from build123d import *

# Parameters (mm, degrees)
F0_R     = 6.25
F1_DEPTH = 8


with BuildPart() as f1:
    # F0 (on Top) → F1 (new body)
    with BuildSketch(Plane.XY):
        Polygon((9.494796, -5.493831), (9.505195, 5.475819), (0.010399, 10.96965), (-9.494796, 5.493831), (-9.505195, -5.475819), (-0.010399, -10.96965), align=None)
        Circle(F0_R, mode=Mode.SUBTRACT)
    extrude(amount=F1_DEPTH)

    # F2 (on Right) → F3 (revolve)
    with BuildSketch(Plane.YZ):
        Polygon((11, 0), (0, 0), (0, -11), (19, -11), (19, -8), align=None)
    revolve(axis=Axis((0, 0, -5.5), (0, 0, 1)))


solid = f1.part
Model file for the job. Use its own axes, mm. A direction names the side the tool comes from. Give positions to 0.01 mm unless a question says otherwise; leave off trailing zeros. Write each loop counter-clockwise with the first axis right and the second up, starting at its lowest first coordinate (ties: lowest second). Pieces come first, ordered by that corner, then holes. Notation, with made-up numbers: M 11,55 L 70,55 A28 cw 70,92 Z; hole C 17,-34 d11. An arc over 180 degrees is marked long. One line per item, written item: value. Start each with the question number.
Q1. Saw through at A-A, the plane z = 2. Write the cut outline in (x, y), plus the area to 3 significant figures.
Q2. Saw through at C-C, the plane z = -9.25. Write the cut outline in (x, y), plus the area to 3 significant figures.
Q3. Probe probe 1 along Y at (x, z) = (0, 4); probe 2 along Z at (x, y) = (-4.5, 10); probe 3 along Y at (x, z) = (4, 3). List the from-to ranges inside material, lowest first. Write a range as [from, to].
Q4. Saw through at D-D, the plane z = -5.5. Write the cut outline in (x, y), plus the area to 3 significant figures.
Q5. Drop flat-ended pins along their axis: pin 1 Ø8 at (y, z) = (6.5, 5) entering from -X; pin 2 Ø4 at (x, y) = (0.5, -0.5) entering from +Z; pin 3 Ø10 at (y, z) = (14.5, -4.5) entering from -X. Give the stop position or say it passes through.
Q6. 3-axis set-ups, long thin cutter, end or side, ignore diameter. For faces 1 (the flat face through (4.676, -8.27, 3.944)), 2 (the flat face through (-4.8, -8.2, 3.9)), 3 (the flat face through (4.8, 8.2, 3.9)), 4 (the cylindrical face through (5.96, 1.88, 3.94)): which of +Z, -Z, +X, -X, +Y, -Y reach the whole face in a straight line?
Q7. Saw through at B-B, the plane y = 0. Write the cut outline in (x, z), plus the area to 3 significant figures.
Output values:
1. outline: M -9.51,-5.48 L -0.01,-10.97 L 9.49,-5.49 L 9.51,5.48 L 0.01,10.97 L -9.49,5.49 Z; hole C 0,0 d12.5
1. area: 190 mm²
2. outline: C 0,0 d38
2. area: 1,130 mm²
3. probe 1: y = [-10.96, -6.25], [6.25, 10.96]
3. probe 2: z = [-11, 0]
3. probe 3: y = [-8.66, -4.8], [4.8, 8.66]
4. outline: C 0,0 d33
4. area: 855 mm²
5. pin 1: stops at x = -9.5
5. pin 2: stops at z = 0
5. pin 3: stops at x = -15.54
6. face 1: +Z, +X, -Y
6. face 2: +Z, -X, -Y
6. face 3: +Z, +X, +Y
6. face 4: +Z
7. outline: M -19,-11 L 19,-11 L 19,-8 L 11,0 L 9.5,0 L 9.5,8 L 6.25,8 L 6.25,0 L -6.25,0 L -6.25,8 L -9.5,8 L -9.5,0 L -11,0 L -19,-8 Z
7. area: 406 mm²
